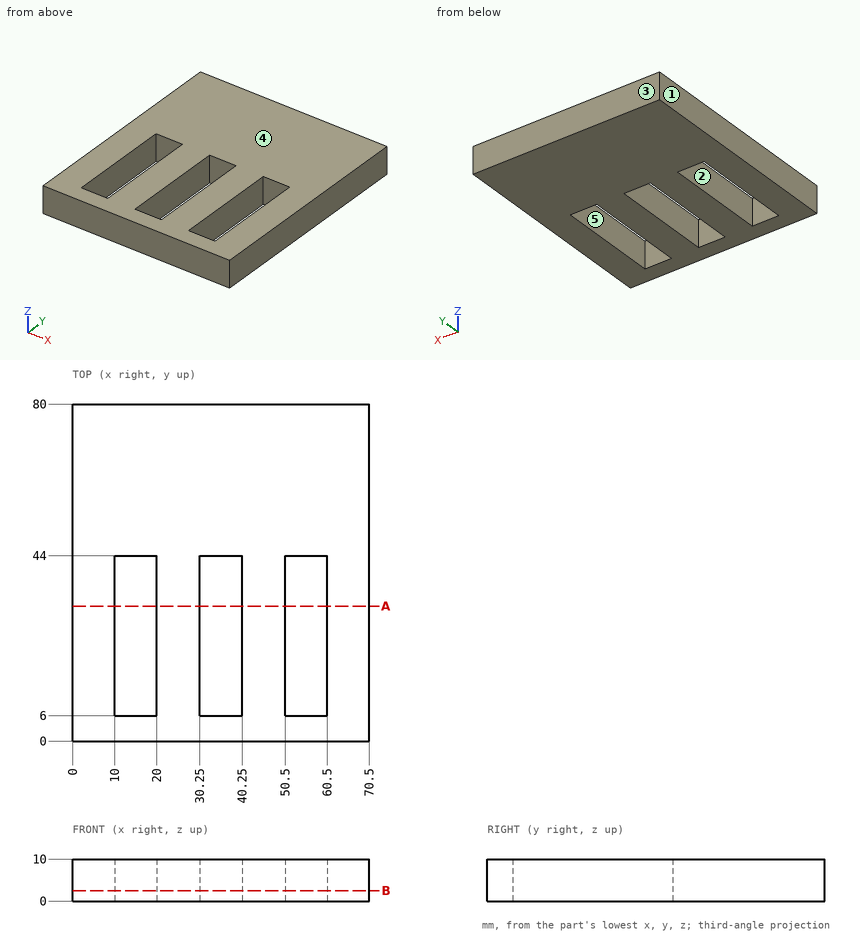
Can you work these out from the drawing? Everything is in mm from the part's minimum corner. A direction names the side the tool comes from. Coordinates: 2 decimals unless noted, no trailing zeros. Loops run counter-clockwise (first coordinate to the right, second up) from the corner with the lowest first, then second, coordinate; pieces in that order, holes last.
1. For the marked faces 4 and 5, which set-ups out of +Z, -Z, +X, -X, +Y, -Y let a thin tool reach every point of the face, with its end or its side?
2. Imagine slicing it at B-B, the plane z = 2.5. Please give me the cut outline in (x, y), and give its area (3 significant figures).
3. Imagine slicing it at A-A, the plane y = 32. Please give me the cut outline in (x, z).
4. I need wall thicknesses on L1, parallel to X at y = 9, z = 9.25; L2, parallel to Y at x = 34, z = 8.25. Which ranges of each line are inside material? Lowest first, please.
5. If we mould it in two halves opening along Y, with no side actions, what happens to the marked faces 1, 2 and 3? For each: pulls with the +Y half, pulls with the -Y half, needs draft (parallel to the pull), parting line crosses it, or undercut.
Taken from the geometry:
1. face 4: +Z, +X, -X, +Y, -Y
1. face 5: +Z, -Z
2. outline: (0, 0) - (70.5, 0) - (70.5, 80) - (0, 80) - close; hole (10, 6) - (20, 6) - (20, 44) - (10, 44) - close; hole (30.25, 6) - (40.25, 6) - (40.25, 44) - (30.25, 44) - close; hole (50.5, 6) - (60.5, 6) - (60.5, 44) - (50.5, 44) - close
2. area: 4,500 mm2
3. outline: (0, 0) - (10, 0) - (10, 10) - (0, 10) - close; (20, 0) - (30.25, 0) - (30.25, 10) - (20, 10) - close; (40.25, 0) - (50.5, 0) - (50.5, 10) - (40.25, 10) - close; (60.5, 0) - (70.5, 0) - (70.5, 10) - (60.5, 10) - close
4. L1: x = 0 to 10, 20 to 30.25, 40.25 to 50.5, 60.5 to 70.5
4. L2: y = 0 to 6, 44 to 80
5. face 1: needs draft
5. face 2: undercut
5. face 3: pulls with the +Y half
